Drawing for the job (mm, zero at the part's lowest x, y, z). Coordinates: 2 decimals unless noted, no trailing zeros. Loops run counter-clockwise (first coordinate to the right, second up) from the corner with the lowest first, then second, coordinate; pieces in that order, holes last. Notation, with made-up numbers: (-38, 11) - (-14, 11) arc R20 ccw to (-14, 46) - close; hole circle Ø10 at (-34.5, 66.25). An arc over 180 degrees is marked (long way). Put each result on its own line as item: value.
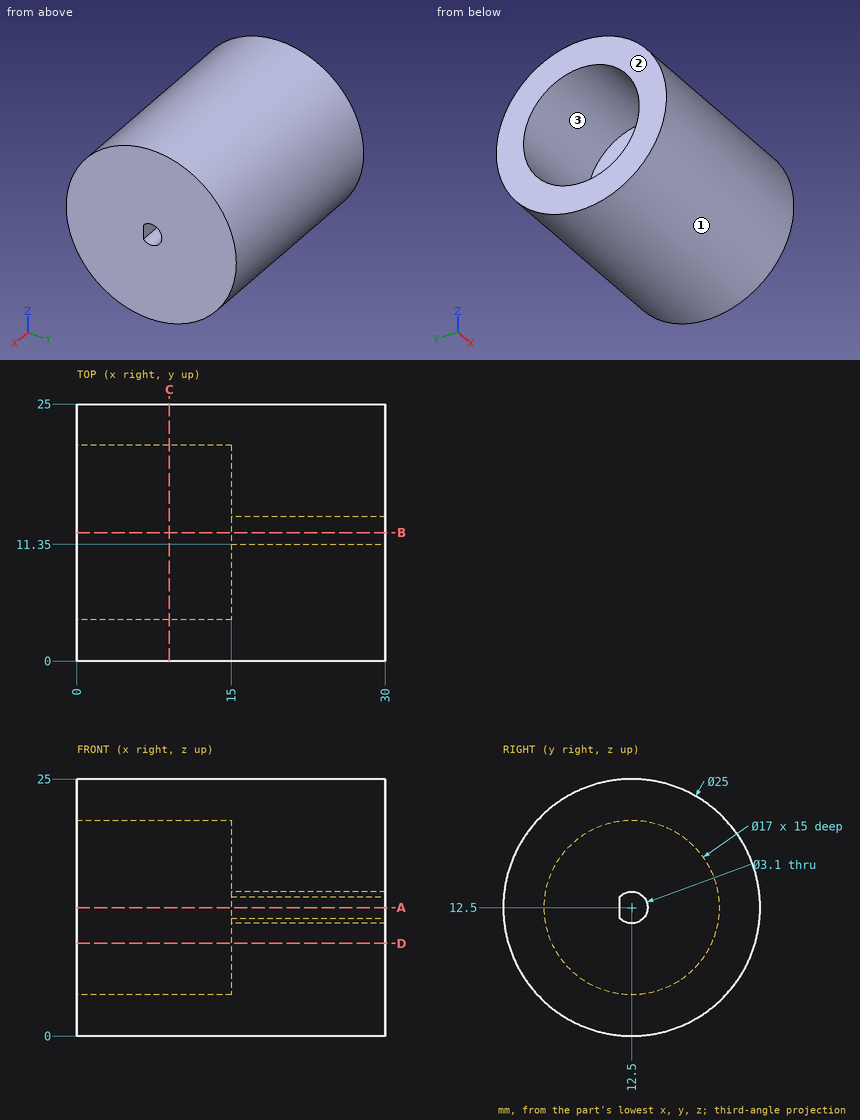
Q1. Slice it at C-C, the plane x = 9. Give the cut face in (y, z), then the cut area to 3 significant figures.
Determined:
outline: circle Ø25 at (12.5, 12.5); hole circle Ø17 at (12.5, 12.5)
area: 264 mm2
Q2. Slice it at D-D, the plane z = 9. Give the cut face in (x, y), then the cut area to 3 significant figures.
Determined:
outline: (0, 0.5) - (30, 0.5) - (30, 24.5) - (0, 24.5) - (0, 20.25) - (15, 20.25) - (15, 4.75) - (0, 4.75) - close
area: 488 mm2
Q3. Mould opens along Z. For the marked faces 1, 2 and 3 say: +Z half, -Z half, draft (parallel to the pull), parting line (faces both ways), or undercut.
Determined:
face 1: parting line
face 2: draft
face 3: undercut
Q4. Slice it at A-A, the plane z = 12.5. Give the cut face in (x, y).
Determined:
outline: (0, 0) - (30, 0) - (30, 11.35) - (15, 11.35) - (15, 4) - (0, 4) - close; (0, 21) - (15, 21) - (15, 14.05) - (30, 14.05) - (30, 25) - (0, 25) - close
Q5. Pin check, flat tips, straight feed: pin 1 Ø12 at (x, y) = (22.5, 21) entering from +Z; pin 2 Ø8 at (x, y) = (13, 18) entering from +Z; pin 3 Ø2 at (y, z) = (14, 7) entering from -X. Stop position of each tip, or through.
Determined:
pin 1: z = 24.75
pin 2: z = 24.91
pin 3: x = 15
Q6. Wall check: L1, parallel to Z at x = 25.5, y = 12.5; L2, parallel to X at y = 7.5, z = 17.25; L3, parallel to Y at x = 8, z = 17.75. Give the ranges that are in metal, low to high. Write a range as from..to.
Determined:
L1: 0..10.95, 14.05..25
L2: 15..30
L3: 1.16..5.82, 19.18..23.84
Q7. Slice it at B-B, the plane y = 12.5. Give the cut face in (x, z).
Determined:
outline: (0, 0) - (30, 0) - (30, 10.95) - (15, 10.95) - (15, 4) - (0, 4) - close; (0, 21) - (15, 21) - (15, 14.05) - (30, 14.05) - (30, 25) - (0, 25) - close
